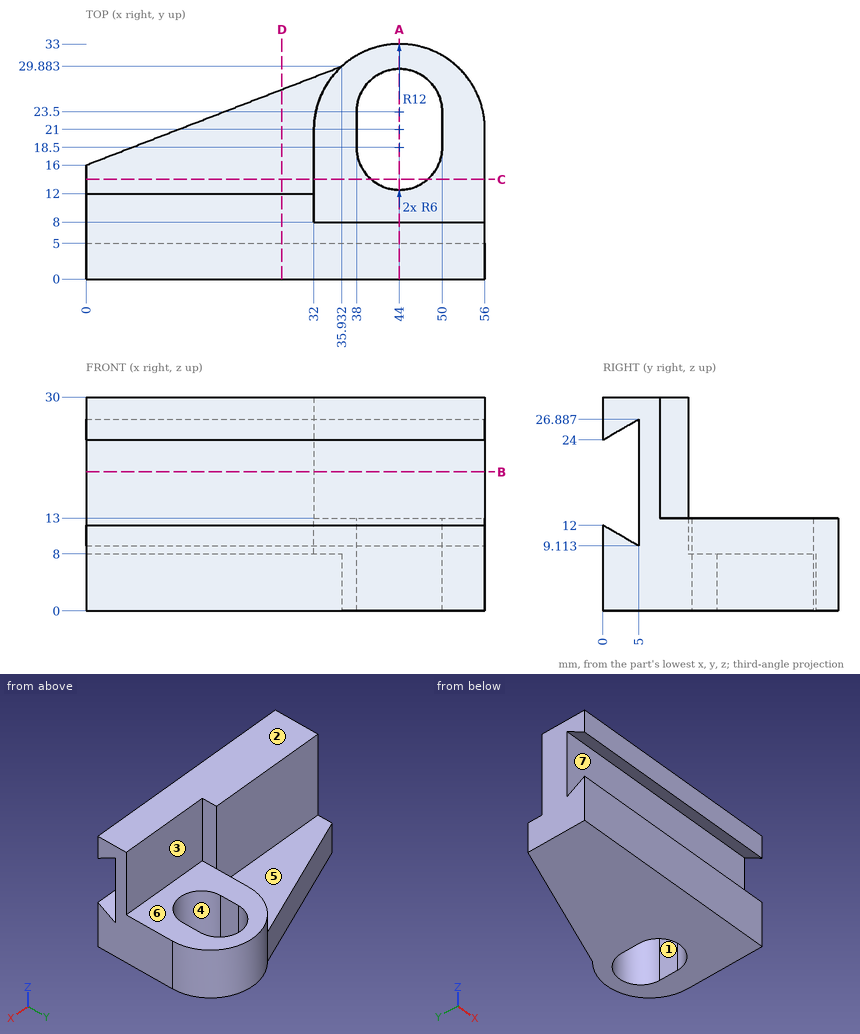
Can you work these out from the drawing? Everything is in mm from the part's minimum corner. A direction names the side the tool comes from. Coordinates: 2 decimals unless noted, no trailing zeros. Write each loop counter-clockwise with the first axis right and the second up, starting at its lowest first coordinate (ties: lowest second). Pieces come first, ordered by that corner, then holes. Notation, with made-up numbers: (7, 48.5) - (59, 48.5) arc R16 cw to (59, 63.5) - close; hole circle Ø10 at (58, 58.5). An arc over 180 degrees is marked (long way). One line per item, written item: value.
1) I need wall thicknesses on line 1 along X through (y, z) = (21.5, 9.25); line 2 along Y through (x, z) = (16.5, 27.75); line 3 along Y through (x, z) = (44.5, 28.75). Which ranges of each line are inside material? Lowest first, please.
Model answer:
line 1: x = 32.01 to 38, 50 to 55.99
line 2: y = 0 to 12
line 3: y = 0 to 8
2) I'm going to push flat-ended pins straight in: P1, Ø7, axis at x = 40, y = 17, coming from the +Z side; P2, Ø8.5, axis at x = 43.5, z = 24, coming from the +Y side; P3, Ø5.5, axis at x = 32, z = 19, coming from the -Y side. Where does each tip first touch, or does it pass through?
Model answer:
P1: stops at z = 13
P2: stops at y = 8
P3: stops at y = 5
3) Suppose I cut it at C-C on y = 14. Write out the boundary of the cut face in (x, z).
Model answer:
outline: (0, 0) - (40.03, 0) - (40.03, 13) - (32, 13) - (32, 8) - (0, 8) - close; (47.97, 0) - (56, 0) - (56, 13) - (47.97, 13) - close
4) Suppose I cut it at A-A on x = 44. Write out the boundary of the cut face in (y, z).
Model answer:
outline: (0, 0) - (12.5, 0) - (12.5, 13) - (8, 13) - (8, 30) - (0, 30) - (0, 24) - (5, 26.89) - (5, 9.11) - (0, 12) - close; (29.5, 0) - (33, 0) - (33, 13) - (29.5, 13) - close
5) Suppose I cut it at B-B on z = 19.5. Write out the boundary of the cut face in (x, y), and give its area (3 significant figures).
Model answer:
outline: (0, 5) - (56, 5) - (56, 8) - (32, 8) - (32, 12) - (0, 12) - close
area: 296 mm²
6) We'd pull the mould along Y, two halves only. Please class the marked faces 1, 2 and 3: pulls with the +Y half, pulls with the -Y half, needs draft (parallel to the pull), parting line crosses it, or undercut.
Model answer:
face 1: undercut
face 2: needs draft
face 3: pulls with the +Y half
7) On a 3-axis mill with a long thin cutter (end or side, diameter ignored), from which of +Z, -Z, +X, -X, +Y, -Y can I reach the whole of each face in a straight line? I mean the marked faces 4, 5, 6 and 7. Say none if no direction works.
Model answer:
face 4: +Z, -Z
face 5: +Z, -X, +Y
face 6: +Z, +X, +Y
face 7: +X, -X
8) Suppose I cut it at D-D on x = 27.5. Write out the boundary of the cut face in (y, z) (1 decimal).
Model answer:
outline: (0, 0) - (26.6, 0) - (26.6, 8) - (12, 8) - (12, 30) - (0, 30) - (0, 24) - (5, 26.9) - (5, 9.1) - (0, 12) - close
